Check sheet for the modelled part. Datum: model origin and axes. Units: mm. A direction names the side the tool comes from. Round coordinates to 2 decimals unless told otherwise and drop trailing zeros. Loops run counter-clockwise (first coordinate to the right, second up) from the corner with the lowest first, then second, coordinate; pieces in that order, holes last. Notation, with made-up numbers: (50.25, -38.75) - (104.25, -38.75) arc R28 ccw to (104.25, -14.75) - close; hole circle Ø6 at (-20.5, 13.25). An arc over 180 degrees is marked (long way). Put each result on its own line as item: value. Start each with the question number.
Item 1: Material ranges on line 1 along Z through (x, y) = (46, 7); line 2 along Z through (x, y) = (5, 7.5); line 3 along X through (y, z) = (11.5, 8.5), recorded low to high.
Item 2: Draft check along Z on faces 1 (the cylindrical face through (46.969, 7.308, 33.863)), 2 (the flat face through (52, 14, 20)), 3 (the conical face through (6.984, 20.364, 24.957)), 4 (the conical face through (45.65, 15.04, 31.89)). Enter one of: pulls with the +Z half, pulls with the -Z half, needs draft (parallel to the pull), parting line crosses it, or undercut.
Item 3: Section check A-A, the plane x = 26. Record the cut outline in (y, z), and give its area (3 significant figures).
Item 4: Gauge pin test, flat ends, axial feed: pin 1 Ø2.5 at (x, y) = (7, 20) entering from +Z; pin 2 Ø5.5 at (x, z) = (6, 8) entering from +Y; pin 3 Ø5 at (x, z) = (6, 32) entering from +Y. Record the tip position at first contact, or that the pin passes through.
Item 5: Section check C-C, the plane y = 8. Give the number of separate pieces and of enclosed holes in the cut face, and give its area (3 significant figures).
Item 6: Tool access check on faces 5 (the cylindrical face through (46.041, 33.874, 0.057)), 6 (the cylindrical face through (40.853, 8.114, 32.883)). Record the directions out of +Z, -Z, +X, -X, +Y, -Y that give a thin tool (end or side, any length) a straight path to the whole face; none if there is none.
Item 7: Section check B-B, the plane z = 17.5. Record the cut outline in (x, y), and give its area (3 significant figures).
from build123d import *

# Parameters (mm, degrees)
ESQUISSE1_W              = 52
ESQUISSE1_H              = 40
ESQUISSE1_R              = 14
BOSS_EXTRU_1_DEPTH       = 40
CHANFREIN1_SIZE          = 12
CONG_1_R                 = 0.2
M5X0_81_D                = 4.2
M5X0_81_DEPTH            = 14
M5X0_81_CSINK_D          = 5.05
M5X0_81_CSINK_ANGLE      = 90
M5X0_81_TIP              = 1.2618073
M5X0_82_AT_2_COUNT       = 2
M5X0_82_AT_2_PITCH       = 38
PATTERN_CIRCULAR_1_COUNT = 2
PATTERN_CIRCULAR_1_ANGLE = 45
PATTERN_CIRCULAR_2_COUNT = 2
PATTERN_CIRCULAR_2_ANGLE = 315


with BuildPart() as part:
    # Esquisse1 → Boss.-Extru.1 (new body)
    with BuildSketch(Plane.XY):
        with Locations((26, 20)):
            Rectangle(ESQUISSE1_W, ESQUISSE1_H)
        with Locations((26, 20)):
            Circle(ESQUISSE1_R, mode=Mode.SUBTRACT)
    extrude(amount=BOSS_EXTRU_1_DEPTH)

    # Chanfrein1
    chanfrein1_edges = [part.edges().sort_by_distance(p)[0] for p in [
        (0, 40, 20),
        (52, 40, 20),
    ]]
    chamfer(chanfrein1_edges, length=CHANFREIN1_SIZE)

    # Cong_1
    cong_1_edges = [part.edges().sort_by_distance(p)[0] for p in [
        (52, 14, 40),
        (12, 20, 0),
        (0, 14, 0),
        (0, 14, 40),
        (0, 28, 20),
        (26, 40, 0),
        (46, 34, 0),
        (6, 34, 0),
        (26, 40, 40),
        (40, 40, 20),
        (12, 40, 20),
        (46, 34, 40),
        (6, 34, 40),
        (52, 28, 20),
        (52, 14, 0),
        (26, 0, 0),
        (26, 0, 40),
        (52, 0, 20),
        (0, 0, 20),
    ]]
    fillet(cong_1_edges, radius=CONG_1_R)

    # M5x0.81
    with Locations(Plane(origin=(0, 0, 0), x_dir=(-1, 0, 0), z_dir=(0, -1, 0))):
        with Locations((-6, -32), (-46, -32), (-46, -8), (-6, -8)):
            CounterSinkHole(M5X0_81_D / 2, M5X0_81_CSINK_D / 2, depth=M5X0_81_DEPTH, counter_sink_angle=M5X0_81_CSINK_ANGLE)
            with Locations((0, 0, -(M5X0_81_DEPTH + M5X0_81_TIP / 2))):  # 118° drill point
                Cone(0, M5X0_81_D / 2, M5X0_81_TIP, mode=Mode.SUBTRACT)

    # Sketch 6 → M5x0.82 (revolve, cut)
    with BuildSketch(Plane(origin=(7, 20, 40), x_dir=(0, -1, 0), z_dir=(1, 0, 0))):
        Polygon((0, 0), (0, 15.2618073), (2.1, 14), (2.1, 0.425), (2.525, 0), align=None)
    m5x0_82 = revolve(axis=Axis((7, 20, 46.35), (0, 0, -1)), mode=Mode.SUBTRACT)

    # M5x0.82 at 2: M5x0.82 ×2
    with Locations(*[(i * M5X0_82_AT_2_PITCH, 0, 0) for i in range(1, M5X0_82_AT_2_COUNT)]):
        add(m5x0_82, mode=Mode.SUBTRACT)

    # Pattern Circular 1: M5x0.82 ×2 about axis
    pattern_circular_1_axis = Axis((26, 20, 0), (0, 0, 1))
    for i in range(1, PATTERN_CIRCULAR_1_COUNT):
        add(m5x0_82.rotate(pattern_circular_1_axis, i * PATTERN_CIRCULAR_1_ANGLE / (PATTERN_CIRCULAR_1_COUNT - 1)), mode=Mode.SUBTRACT)

    # Pattern Circular 1 copy 1 sketch → Pattern Circular 1 copy 1 (revolve, cut)
    with BuildSketch(Plane(origin=(39.435028843, 33.435028843, 40), x_dir=(0.7071067811865488, -0.7071067811865462, 0), z_dir=(0.7071067811865462, 0.7071067811865488, 0))):
        Polygon((0, 0), (0, 15.2618073), (2.1, 14), (2.1, 0.425), (2.525, 0), align=None)
    revolve(axis=Axis((39.435028843, 33.435028843, 46.35), (0, 0, -1)), mode=Mode.SUBTRACT)

    # Pattern Circular 2: M5x0.82 ×2 about axis
    pattern_circular_2_axis = Axis((26, 20, 0), (0, 0, 1))
    for i in range(1, PATTERN_CIRCULAR_2_COUNT):
        add(m5x0_82.rotate(pattern_circular_2_axis, i * PATTERN_CIRCULAR_2_ANGLE / (PATTERN_CIRCULAR_2_COUNT - 1)), mode=Mode.SUBTRACT)

    # Pattern Circular 2 copy 1 sketch → Pattern Circular 2 copy 1 (revolve, cut)
    with BuildSketch(Plane(origin=(39.435028843, 6.564971157, 40), x_dir=(-0.7071067811865389, -0.7071067811865561, 0), z_dir=(0.7071067811865561, -0.7071067811865389, 0))):
        Polygon((0, 0), (0, 15.2618073), (2.1, 14), (2.1, 0.425), (2.525, 0), align=None)
    revolve(axis=Axis((39.435028843, 6.564971157, 46.35), (0, 0, -1)), mode=Mode.SUBTRACT)


solid = part.part
Check result:
1. line 1: 0 to 5.9, 10.1 to 29.9, 34.1 to 40
1. line 2: 0 to 6.15, 9.85 to 30.15, 33.85 to 40
1. line 3: 0 to 3.96, 8.04 to 14.88, 37.12 to 43.96, 48.04 to 52
2. face 1: undercut
2. face 2: needs draft
2. face 3: pulls with the +Z half
2. face 4: undercut
3. outline: (0, 0.2) arc R0.2 ccw to (0.2, 0) - (5.8, 0) arc R0.2 ccw to (6, 0.2) - (6, 40) - (0.2, 40) arc R0.2 ccw to (0, 39.8) - close; (34, 0.2) arc R0.2 ccw to (34.2, 0) - (39.8, 0) arc R0.2 ccw to (40, 0.2) - (40, 39.8) arc R0.2 ccw to (39.8, 40) - (34, 40) - close
3. area: 480 mm²
4. pin 1: z = 25.49
4. pin 2: y = 36.75
4. pin 3: y = 36.5
5. separate pieces: 2
5. enclosed holes: 4
5. area: 1,360 mm²
6. face 5: -Z, +X, +Y
6. face 6: +Z
7. outline: (0, 0.2) arc R0.2 ccw to (0.2, 0) - (51.8, 0) arc R0.2 ccw to (52, 0.2) - (52, 27.92) arc R0.2 ccw to (51.94, 28.06) - (40.06, 39.94) arc R0.2 ccw to (39.92, 40) - (12.08, 40) arc R0.2 ccw to (11.94, 39.94) - (0.06, 28.06) arc R0.2 ccw to (0, 27.92) - close; hole circle Ø28 at (26, 20)
7. area: 1,320 mm²
